Build history of the part. All positions in model axes, mm. Round coordinates to 2 decimals unless told otherwise and drop trailing zeros. Write each loop counter-clockwise with the first axis right and the second up, starting at its lowest first coordinate (ties: lowest second). Pieces come first, ordered by that corner, then holes. Notation, with made-up numbers: M -22,-6.75 L 21,-6.75 A25 ccw 21,28.25 Z; hole C 58,-14 d10. An arc over 180 degrees is marked long. Write item = value, one per line. Start each with the question number.
Q1. Band-saw the part on B-B on x = 0. Write the cut outline in (y, z), plus the area to 3 significant figures.
Q2. Probe L1, parallel to Z at x = -0.25, y = 2.5; L2, parallel to X at y = 2.75, z = 69.5; L3, parallel to Z at x = -1, y = -4.25. List the from-to ranges inside material, lowest first.
Q3. Band-saw the part on A-A on z = 5.5. Write the cut outline in (x, y), plus the area to 3 significant figures.
Q4. Drop a flat-ended pin along its axis: P1, Ø3.5, axis at x = 0, z = 15.5, coming from the -Y side. Give the stop position or say it passes through.
Q5. Band-saw the part on C-C on y = -3.25. Write the cut outline in (x, z).
```python
from build123d import *

# Parameters (mm, degrees)
SKETCH1_W           = 13
SKETCH1_H           = 13
BOSS_EXTRUDE1_DEPTH = 75
SKETCH2_R           = 2
CUT_EXTRUDE1_DEPTH  = 75


with BuildPart() as part:
    # Sketch1 → Boss-Extrude1 (new body)
    with BuildSketch(Plane.XY):
        Rectangle(SKETCH1_W, SKETCH1_H)
    extrude(amount=BOSS_EXTRUDE1_DEPTH)

    # Sketch2 → Cut-Extrude1 (cut)
    with BuildSketch(Plane(origin=(0, 6.5, 0), x_dir=(1, 0, 0), z_dir=(0, 1, 0))):
        with Locations(Location((0, -69.5, 0), (0, 0, 270))):
            Circle(SKETCH2_R)
        with Locations(Location((0, -59.5, 0), (0, 0, 270))):
            Circle(SKETCH2_R)
        with Locations(Location((0, -5.5, 0), (0, 0, 270))):
            Circle(SKETCH2_R)
        with Locations(Location((0, -15.5, 0), (0, 0, 270))):
            Circle(SKETCH2_R)
    extrude(amount=-CUT_EXTRUDE1_DEPTH, mode=Mode.SUBTRACT)


solid = part.part
```
Conclusion:
q1.outline = M -6.5,0 L 6.5,0 L 6.5,3.5 L -6.5,3.5 Z; M -6.5,7.5 L 6.5,7.5 L 6.5,13.5 L -6.5,13.5 Z; M -6.5,17.5 L 6.5,17.5 L 6.5,57.5 L -6.5,57.5 Z; M -6.5,61.5 L 6.5,61.5 L 6.5,67.5 L -6.5,67.5 Z; M -6.5,71.5 L 6.5,71.5 L 6.5,75 L -6.5,75 Z
q1.area = 767 mm^2
q2.L1 = 0 to 3.52, 7.48 to 13.52, 17.48 to 57.52, 61.48 to 67.52, 71.48 to 75
q2.L2 = -6.5 to -2, 2 to 6.5
q2.L3 = 0 to 3.77, 7.23 to 13.77, 17.23 to 57.77, 61.23 to 67.77, 71.23 to 75
q3.outline = M -6.5,-6.5 L -2,-6.5 L -2,6.5 L -6.5,6.5 Z; M 2,-6.5 L 6.5,-6.5 L 6.5,6.5 L 2,6.5 Z
q3.area = 117 mm^2
q4.P1 = through
q5.outline = M -6.5,0 L 6.5,0 L 6.5,75 L -6.5,75 Z; hole C 0,5.5 d4; hole C 0,15.5 d4; hole C 0,59.5 d4; hole C 0,69.5 d4
